Autodesk Inventor part; units mm, degrees
ref_plane "YZ Plane" through (0, 0, 0) normal (1, 0, 0) x (0, 1, 0)
ref_plane "XZ Plane" through (0, 0, 0) normal (0, 1, 0) x (-1, 0, 0)
ref_plane "XY Plane" through (0, 0, 0) normal (0, 0, 1) x (1, 0, 0)
sketch "Sketch1" plane through (0, 0, 0) normal (0, 0, 1) x (1, 0, 0)
  circle A0 centre (0, 0) radius 3.429
  dimension "d0" = 6.858
extrude "Extrusion1" add sketch "Sketch1" along normal blind 4.064
sketch "Sketch2" plane through (0, 0, 4.064) normal (0, 0, 1) x (1, 0, 0)
  line L0 (-1.0514, 1.7804) -> (1.0162, 1.8008)
  line L1 (1.0162, 1.8008) -> (2.0676, 0.0204)
  line L2 (2.0676, 0.0204) -> (1.0514, -1.7804)
  line L3 (1.0514, -1.7804) -> (-1.0162, -1.8008)
  line L4 (-1.0162, -1.8008) -> (-2.0676, -0.0204)
  line L5 (-2.0676, -0.0204) -> (-1.0514, 1.7804)
  point P0 (0, 0)
  point P1 (0, 0)
  dimension "d3" = 3.5814
extrude "Extrusion2" cut sketch "Sketch2" against normal blind 2.54
chamfer "Chamfer1" distance 0.254 angle 45 1 edges at (-3.429, 0, 4.064)
sketch "Sketch3" plane through (0, 0, 0) normal (0, 0, -1) x (-1, 0, 0)
  circle A0 centre (0, 0) radius 2.032
  dimension "d9" = 4.064
extrude "Extrusion3" add sketch "Sketch3" along normal blind 12.7
thread "Thread1"
properties part number "8-32 UNC Bolt" material "Stainless Steel"
The listing builds one solid part. Answer for the finished solid, in the listing's coordinates (mm). A direction names the side the tool comes from. Give positions to 0.01 mm unless a question says otherwise; leave off trailing zeros. Write each loop counter-clockwise with the first axis right and the second up, starting at its lowest first coordinate (ties: lowest second). Pieces come first, ordered by that corner, then holes.
1) Given P1, Ø1.1, axis at x = 0, y = 1, coming from the +Z side; P2, Ø1.5, axis at x = -1.5, z = -8.5, coming from the +Y side; P3, Ø1, axis at x = -1.5, z = -5.5, coming from the +Y side, each flat-ended and moving along its own axis, determine where each tip first touches the part or whether it passes through.
2) For a pull along Y with two mould halves and no side action, classify faces 1 (the face through (-0.74, 3.35, 1.88)), 2 (the face through (-1.567, 0.867, 2.812)), 3 (the face through (0, 0, -12.7)) as pulls with the +Y half, pulls with the -Y half, needs draft (parallel to the pull), parting line crosses it, or undercut.
3) Section B-B (z = -7.5) is taken. Write down the section's boundary in (x, y).
4) Find the intervals of material crossed by L1, parallel to Z at x = 0.5, y = 1.75; L2, parallel to Z at x = -1.75, y = -2.25; L3, parallel to X at y = -1.5, z = 3, in increasing order.
5) Section A-A (x = 0) is taken. Write down the section's boundary in (y, z) (3 decimals), and give its area (3 significant figures).
6) A tool of negligible diameter and unlimited length cuts with its end or side. For faces 4 (the face through (0, -2.2, 0)), 5 (the face through (0, -2, 4.064)), 6 (the face through (1.535, 0.923, 2.812)), from which of +Z, -Z, +X, -X, +Y, -Y can it reach the whole face along a straight path? Write none if from no direction.
Response:
1. P1: stops at z = 1.52
1. P2: stops at y = 1.89
1. P3: stops at y = 1.77
2. face 1: parting line crosses it
2. face 2: undercut
2. face 3: needs draft
3. outline: circle Ø4.06 at (0, 0)
4. L1: z = -12.7 to 1.52
4. L2: z = 0 to 4.06
4. L3: x = -3.08 to -1.19, 1.21 to 3.08
5. outline: (-3.429, 0) - (-2.032, 0) - (-2.032, -12.7) - (2.032, -12.7) - (2.032, 0) - (3.429, 0) - (3.429, 3.81) - (3.175, 4.064) - (1.791, 4.064) - (1.791, 1.524) - (-1.791, 1.524) - (-1.791, 4.064) - (-3.175, 4.064) - (-3.429, 3.81) - close
5. area: 70.3 mm2
6. face 4: -Z
6. face 5: +Z, +X, -X, +Y, -Y
6. face 6: +Z
